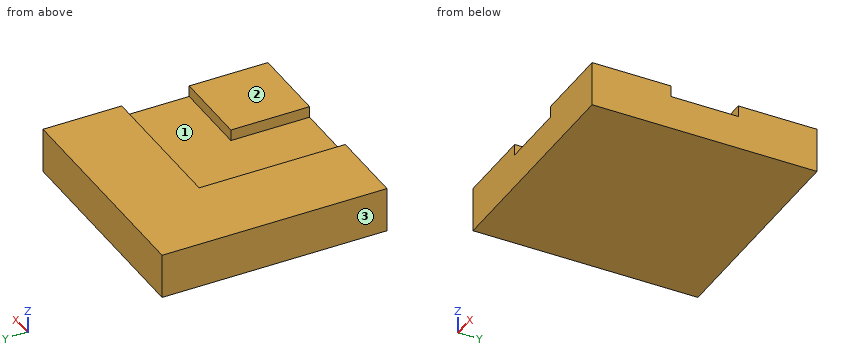
Solid Edge part; units mm, degrees
sketch "Sketch1" plane through (0, 0, 0) normal (0, 0, 1) x (1, 0, 0)
  line L0 (-10, -10) -> (10, -10)
  line L1 (10, -10) -> (10, 10)
  line L2 (10, 10) -> (-10, 10)
  line L3 (-10, 10) -> (-10, -10)
extrude "Protrusion1" add sketch "Sketch1" along normal blind 3
sketch "Sketch2" plane through (0, 0, 3) normal (0, 0, 1) x (1, 0, 0)
  line L0 (-10, -10) -> (-5, -10)
  line L1 (-5, -10) -> (-5, 10)
  line L2 (-5, 10) -> (-10, 10)
  line L3 (-10, 10) -> (-10, -10)
extrude "Extrusionsausprägung_2" add sketch "Sketch2" along normal blind 1
sketch "Sketch3" plane through (2.5, 0, 3) normal (0, 0, 1) x (1, 0, 0)
  line L0 (-7.5, 10) -> (7.5, 10)
  line L1 (7.5, 10) -> (7.5, 5)
  line L2 (7.5, 5) -> (-7.5, 5)
  line L3 (-7.5, 5) -> (-7.5, 10)
extrude "Extrusionsausprägung_3" add sketch "Sketch3" along normal blind 1
sketch "Sketch4" plane through (2.5, -2.5, 3) normal (0, 0, 1) x (1, 0, 0)
  line L0 (7.5, -7.5) -> (7.5, -2.5)
  line L1 (7.5, -2.5) -> (2.5, -2.5)
  line L2 (2.5, -2.5) -> (2.5, -7.5)
  line L3 (2.5, -7.5) -> (7.5, -7.5)
extrude "Extrusionsausprägung_4" add sketch "Sketch4" along normal blind 1
sketch "Sketch5" plane through (2.5, -2.5, 3) normal (0, 0, 1) x (1, 0, 0)
  line L0 (2.5, -7.5) -> (1.5, -7.5)
  line L1 (1.5, -7.5) -> (1.5, -2.4982)
  line L2 (1.5, -1.5) -> (1.5, -2.4982)
  line L3 (7.5, -1.5) -> (1.5, -1.5)
  line L4 (7.5, -2.5) -> (7.5, -1.5)
  line L5 (7.5, -2.5) -> (2.5, -2.5)
  line L6 (2.5, -2.5) -> (2.5, -7.5)
extrude "Extrusionsausprägung_5" add sketch "Sketch5" along normal blind 1
sketch "Sketch6" plane through (2.5, -2.5, 3) normal (0, 0, 1) x (1, 0, 0)
  line L0 (-7.5, -7.5) -> (-6.5, -7.5)
  line L1 (-6.5, -7.5) -> (-6.5, 6.5)
  line L2 (-6.5, 6.5) -> (7.5, 6.5)
  line L3 (7.5, 6.5) -> (7.5, 7.5)
  line L4 (7.5, 7.5) -> (-7.5, 7.5)
  line L5 (-7.5, 7.5) -> (-7.5, -7.5)
extrude "Extrusionsausprägung_6" add sketch "Sketch6" along normal blind 1
sketch "Sketch7" plane through (3, -3, 3) normal (0, 0, 1) x (1, 0, 0)
  line L0 (-7, -7) -> (-6, -7)
  line L1 (-6, -7) -> (-6, 6)
  line L2 (-6, 6) -> (7, 6)
  line L3 (7, 6) -> (7, 7)
  line L4 (7, 7) -> (-7, 7)
  line L5 (-7, 7) -> (-7, -7)
extrude "Extrusionsausprägung_7" add sketch "Sketch7" along normal blind 1
sketch "Sketch8" plane through (3.5, -3.5, 3) normal (0, 0, 1) x (1, 0, 0)
  line L0 (0.5, -6.5) -> (-0.5, -6.5)
  line L1 (-0.5, -6.5) -> (-0.5, 0.5)
  line L2 (-0.5, 0.5) -> (6.5, 0.5)
  line L3 (6.5, 0.5) -> (6.5, -0.5)
  line L4 (6.5, -0.5) -> (0.5, -0.5)
  line L5 (0.5, -0.5) -> (0.5, -6.5)
extrude "Extrusionsausprägung_8" add sketch "Sketch8" along normal blind 1
Geometry check sheet. Reference: the model listing, model coordinates, mm. Face numbers are marked on the shaded views. Give positions to 0.01 mm unless a question says otherwise; leave off trailing zeros. Write each loop counter-clockwise with the first axis right and the second up, starting at its lowest first coordinate (ties: lowest second). Pieces come first, ordered by that corner, then holes.
1) Cross-section at B-B (x = 3.75). Record the boundary of the cut face in (y, z), plus the area to 3 significant figures.
Values follow:
outline: (-10, 0) - (10, 0) - (10, 4) - (3, 4) - (3, 3) - (-3, 3) - (-3, 4) - (-10, 4) - close
area: 74.0 mm2
2) Release check for a two-part mould opening along X. For the marked faces 1, 2 and 3 record: released by +X, released by -X, zero draft, split by the parting line, or undercut.
Values follow:
face 1: undercut
face 2: zero draft
face 3: released by -X
3) Thickness scan on line 1 (X direction, y = -7.75, z = 3.3); line 2 (Y direction, x = 0.75, z = 3.55). Record the ranges inside material, lowest first.
Values follow:
line 1: x = -10 to -3, 3 to 10
line 2: y = 3 to 10
4) Cross-section at C-C (y = 2.5). Record the boundary of the cut face in (x, z), plus the area to 3 significant figures.
Values follow:
outline: (-10, 0) - (10, 0) - (10, 3) - (-3, 3) - (-3, 4) - (-10, 4) - close
area: 67.0 mm2
5) Go/stop test with a flat-tipped pin: pin 1 Ø2 at (x, y) = (0.5, -2.5) entering from +Z. Record where the tip stops, or that it passes through.
Values follow:
pin 1: stops at z = 3
6) Cross-section at A-A (z = 3.75). Record the boundary of the cut face in (x, y).
Values follow:
outline: (-10, -10) - (-3, -10) - (-3, 3) - (10, 3) - (10, 10) - (-10, 10) - close; (3, -10) - (10, -10) - (10, -3) - (3, -3) - close
